CAD build for the part. Positions are in the model's coordinates, mm. Round coordinates to 2 decimals unless told otherwise and drop trailing zeros. Loops run counter-clockwise (first coordinate to the right, second up) from the corner with the lowest first, then second, coordinate; pieces in that order, holes last.
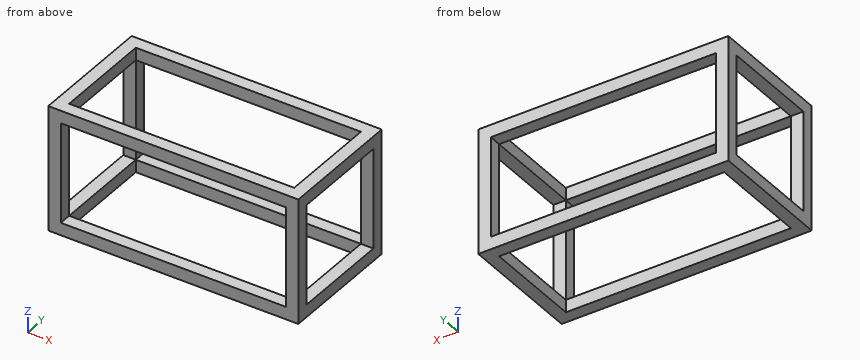
from build123d import *

# Parameters (mm, degrees)
SKETCH1_W           = 100
SKETCH1_H           = 50
SKETCH1_W_2         = 90
SKETCH1_H_2         = 40
BOSS_EXTRUDE1_DEPTH = 50
SKETCH2_W           = 40
SKETCH2_H           = 40
CUT_EXTRUDE1_DEPTH  = 101
SKETCH3_W           = 90
SKETCH3_H           = 40
CUT_EXTRUDE2_DEPTH  = 51


with BuildPart() as part:
    # Sketch1 → Boss-Extrude1 (new body)
    with BuildSketch(Plane(origin=(0, 0, 0), x_dir=(1, 0, 0), z_dir=(0, 1, 0))):
        with Locations((50, 25)):
            Rectangle(SKETCH1_W, SKETCH1_H)
        with Locations((50, 25)):
            Rectangle(SKETCH1_W_2, SKETCH1_H_2, mode=Mode.SUBTRACT)
    extrude(amount=BOSS_EXTRUDE1_DEPTH)

    # Sketch2 → Cut-Extrude1 (cut, through all)
    with BuildSketch(Plane(origin=(100, 0, 0), x_dir=(0, 0, -1), z_dir=(1, 0, 0))):
        with Locations((25, 25)):
            Rectangle(SKETCH2_W, SKETCH2_H)
    extrude(amount=-CUT_EXTRUDE1_DEPTH, mode=Mode.SUBTRACT)

    # Sketch3 → Cut-Extrude2 (cut, through all)
    with BuildSketch(Plane.XY):
        with Locations((50, 25)):
            Rectangle(SKETCH3_W, SKETCH3_H)
    extrude(amount=-CUT_EXTRUDE2_DEPTH, mode=Mode.SUBTRACT)


solid = part.part
Item 1: Cut at D-D (y = 47.5). List the corners of the cut face in (x, z), plus the area to 3 significant figures.
Verdict:
outline: (0, -50) - (100, -50) - (100, 0) - (0, 0) - close; hole (5, -45) - (95, -45) - (95, -5) - (5, -5) - close
area: 1,400 mm2
Item 2: Cut at A-A (z = -47). List the corners of the cut face in (x, y).
Verdict:
outline: (0, 0) - (100, 0) - (100, 50) - (0, 50) - close; hole (5, 5) - (95, 5) - (95, 45) - (5, 45) - close
Item 3: Cut at C-C (y = 11.5). List the corners of the cut face in (x, z), plus the area to 3 significant figures.
Verdict:
outline: (0, -50) - (5, -50) - (5, -45) - (0, -45) - close; (0, -5) - (5, -5) - (5, 0) - (0, 0) - close; (95, -50) - (100, -50) - (100, -45) - (95, -45) - close; (95, -5) - (100, -5) - (100, 0) - (95, 0) - close
area: 100 mm2
Item 4: Wall check: L1, parallel to Y at x = 96.5, z = -41; L2, parallel to X at y = 46, z = -29.5; L3, parallel to Z at x = 89.5, y = 3. Give the ranges that are in metal, low to high.
Verdict:
L1: y = 0 to 5, 45 to 50
L2: x = 0 to 5, 95 to 100
L3: z = -50 to -45, -5 to 0
Item 5: Flat gauge pin, fed straight in: P1, Ø1.5, axis at x = 46.5, z = -1.5, coming from the -Y side. Where does the tip first touch, or does it go through?
Verdict:
P1: stops at y = 0
Item 6: Cut at B-B (x = 60.5). List the corners of the cut face in (y, z).
Verdict:
outline: (0, -50) - (5, -50) - (5, -45) - (0, -45) - close; (0, -5) - (5, -5) - (5, 0) - (0, 0) - close; (45, -50) - (50, -50) - (50, -45) - (45, -45) - close; (45, -5) - (50, -5) - (50, 0) - (45, 0) - close
